Source: CAD feature listing. Evaluate the final solid. Frame: model axes, mm. Round coordinates to 2 decimals unless told otherwise and drop trailing zeros. Write each loop counter-clockwise with the first axis right and the second up, starting at its lowest first coordinate (ties: lowest second). Pieces come first, ordered by that corner, then holes.
from build123d import *

# Parameters (mm, degrees)
SKETCH1_R           = 2.54
BOSS_EXTRUDE1_DEPTH = 0.8128
SKETCH2_R           = 2.54
CUT_EXTRUDE1_DEPTH  = 118.606454516
SKETCH3_R           = 2.54
CUT_EXTRUDE2_DEPTH  = 118.606454516
SKETCH5_R           = 2.54
CUT_EXTRUDE3_DEPTH  = 2.54


with BuildPart() as part:
    # Sketch1 → Boss-Extrude1 (new body)
    with BuildSketch(Plane(origin=(0, 0, 0), x_dir=(1, 0, 0), z_dir=(0, 1, 0))):
        Polygon((0, 88.9), (-76.989658396, 44.45), (-76.989658396, -44.45), (0, -88.9), (76.989658396, -44.45), (76.989658396, 44.45), align=None)
        with Locations(Location((13.322783942, -73.875738686, 0), (0, 0, 270))):
            Circle(SKETCH1_R, mode=Mode.SUBTRACT)
        with Locations(Location((24.32130657, -67.525738686, 0), (0, 0, 270))):
            Circle(SKETCH1_R, mode=Mode.SUBTRACT)
        with Locations(Location((-70.639658396, 12.7, 0), (0, 0, 270))):
            Circle(SKETCH1_R, mode=Mode.SUBTRACT)
        with Locations(Location((-70.639658396, 25.4, 0), (0, 0, 270))):
            Circle(SKETCH1_R, mode=Mode.SUBTRACT)
        with Locations(Location((46.318351826, 54.825738686, 0), (0, 0, 270))):
            Circle(SKETCH1_R, mode=Mode.SUBTRACT)
        with Locations(Location((57.316874454, 48.475738686, 0), (0, 0, 270))):
            Circle(SKETCH1_R, mode=Mode.SUBTRACT)
    extrude(amount=BOSS_EXTRUDE1_DEPTH)

    # Sketch2 → Cut-Extrude1 (cut, through all)
    with BuildSketch(Plane(origin=(0, 0.8128, 0), x_dir=(1, 0, 0), z_dir=(0, 1, 0))):
        with Locations(Location((-49.850334746, 36.846687445, 0), (0, 0, 270))):
            Circle(SKETCH2_R)
        with Locations(Location((-25.4, -43.994090512, 0), (0, 0, 270))):
            Circle(SKETCH2_R)
        with Locations(Location((32.385, 56.092465403, 0), (0, 0, 270))):
            Circle(SKETCH2_R)
        with Locations(Location((56.835334746, -24.748312555, 0), (0, 0, 270))):
            Circle(SKETCH2_R)
    extrude(amount=-CUT_EXTRUDE1_DEPTH, mode=Mode.SUBTRACT)

    # Sketch3 → Cut-Extrude2 (cut, through all)
    with BuildSketch(Plane(origin=(0, 0.8128, 0), x_dir=(1, 0, 0), z_dir=(0, 1, 0))):
        with Locations(Location((-35.319829198, -61.175738686, 0), (0, 0, 270))):
            Circle(SKETCH3_R)
        with Locations(Location((-28.969829198, -50.177216058, 0), (0, 0, 270))):
            Circle(SKETCH3_R)
    extrude(amount=-CUT_EXTRUDE2_DEPTH, mode=Mode.SUBTRACT)

    # Sketch5 → Cut-Extrude3 (cut)
    with BuildSketch(Plane(origin=(0, 0.8128, 0), x_dir=(1, 0, 0), z_dir=(0, 1, 0))):
        with Locations(Location((-2.3169441, -57.353036215, 0), (0, 0, 270))):
            Circle(SKETCH5_R)
        with Locations(Location((-12.222931679, -74.510738686, 0), (0, 0, 270))):
            Circle(SKETCH5_R)
        with Locations(Location((-58.416726717, -47.840738686, 0), (0, 0, 270))):
            Circle(SKETCH5_R)
        with Locations(Location((-48.510714297, -30.683050557, 0), (0, 0, 270))):
            Circle(SKETCH5_R)
    extrude(amount=-CUT_EXTRUDE3_DEPTH, mode=Mode.SUBTRACT)


solid = part.part
1) Section query A-A on z = -12.7. Return the cut outline in (x, y), then the cut area to 3 significant figures.
Taken from the geometry:
outline: (-76.99, 0) - (-73.18, 0) - (-73.18, 0.81) - (-76.99, 0.81) - close; (-68.1, 0) - (76.99, 0) - (76.99, 0.81) - (-68.1, 0.81) - close
area: 121 mm2
2) Material intervals for line 1 (X direction, y = 0.7, z = -55.5); line 2 (X direction, y = 0.3, z = 73.5); line 3 (X direction, y = 0.25, z = 45), sorted ascending.
Taken from the geometry:
line 1: x = -57.85 to 29.92, 34.85 to 43.87, 48.77 to 57.85
line 2: x = -26.67 to -14.55, -9.89 to 10.81, 15.83 to 26.67
line 3: x = -76.04 to -27.73, -23.07 to 76.04
3) Pull-direction query (Z, two-part tool) for faces 1 (the face through (-1, 0.813, -1)), 2 (the face through (-73.12, 0.4, -13.25)), 3 (the face through (-39.034, 0.401, 66.364)); classes: released by +Z, released by -Z, zero draft, split by the parting line, or undercut.
Taken from the geometry:
face 1: zero draft
face 2: undercut
face 3: released by +Z
4) Section query C-C on x = 52. Return the cut outline in (y, z).
Taken from the geometry:
outline: (0, -58.88) - (0.81, -58.88) - (0.81, 58.88) - (0, 58.88) - close
5) Section query B-B on y = 0.2. State how many separate pieces and enclosed holes the cut face has, then the cut area to 3 significant figures.
Taken from the geometry:
separate pieces: 1
enclosed holes: 16
area: 20,200 mm2
6) Contact query for a flat-ended pin moving along its axis: P1, Ø10, axis at x = -53, z = 66, coming from the -Y side. Output: stop coordinate, or through.
Taken from the geometry:
P1: passes through
